Geometry: final body of the model. Coordinates: model frame, mm. A direction names the side the tool comes from. Round coordinates to 2 decimals unless told otherwise and drop trailing zeros. Write each loop counter-clockwise with the first axis right and the second up, starting at its lowest first coordinate (ties: lowest second). Pieces come first, ordered by that corner, then holes. Notation, with made-up numbers: M -1.5,67 L 36.5,67 A28 ccw 36.5,103 Z; hole C 1,-10.75 d7. An arc over 180 degrees is marked long. Use one line per item in the form item = value. Start each with the question number.
Item 1: Pull-direction query (Y, two-part tool) for faces 1 (the flat face through (-28.975, 8.916, 5.105)), 2 (the cylindrical face through (-23.116, 6.452, 0.105)), 3 (the flat face through (-27, 0, 2)), 4 (the cylindrical face through (23.116, 6.452, 0.105)); classes: pulls with the +Y half, pulls with the -Y half, needs draft (parallel to the pull), parting line crosses it, or undercut.
Item 2: Reachability of faces 5 (the flat face through (0, 22, -4.5)), 6 (the flat face through (-24.22, 8.84, 1.77)), 7 (the cylindrical face through (-17.81, 15.51, 4.05)), 8 (the flat face through (27, 0, 2)) from +Z, -Z, +X, -X, +Y, -Y: full face, straight path, thin tool, end or side. Return the list, or none.
Item 3: Ray query, probe 1 along Z at (x, y) = (14.5, 15.25); probe 2 along X at (y, z) = (1, 0); probe 3 along X at (y, z) = (5.5, 5). Return the intervals inside material, ascending.
Item 4: Section query B-B (x = 0). Return loops of the section in (y, z).
Item 5: Pin query (flat end, axial travel): pin 1 Ø3 at (y, z) = (5.5, -2.5) entering from -X; pin 2 Ø4.5 at (x, z) = (30.5, 2) entering from +Y; pin 3 Ø2 at (y, z) = (11, 0.5) entering from +X. Return the tip coordinate at first contact, or that it passes through.
Item 6: Section query A-A (z = -6). Return loops of the section in (x, y).
Item 7: Section query D-D (y = 22). Return loops of the section in (x, z), and give its area (3 significant figures).
Item 8: Section query C-C (y = 7.75). Return loops of the section in (x, z), and give its area (3 significant figures).
from build123d import *

# Parameters (mm, degrees)
SALIENTE_EXTRUIR1_DEPTH = 7.5
SALIENTE_EXTRUIR2_DEPTH = 7.5
CROQUIS3_R              = 2.25
CORTAR_EXTRUIR1_DEPTH   = 46.436769251
CROQUIS4_R              = 4.5
CORTAR_EXTRUIR2_DEPTH   = 44.789268092
CORTAR_EXTRUIR3_DEPTH   = 48.257274572
CORTAR_EXTRUIR4_DEPTH   = 15


with BuildPart() as part:
    # Croquis1 → Saliente-Extruir1 (new, symmetric)
    with BuildSketch(Plane.XY):
        with BuildLine():
            Line((-26, 0), (-21, 0))
            ThreePointArc((-21, 0), (0, 21), (21, 0))
            Line((21, 0), (26, 0))
            ThreePointArc((26, 0), (0, 26), (-26, 0))
        make_face()
    extrude(amount=SALIENTE_EXTRUIR1_DEPTH, both=True)

    # Croquis2 → Saliente-Extruir2 (add, symmetric)
    with BuildSketch(Plane.XY):
        with BuildLine():
            Line((26, 0), (36.5, 0))
            Line((36.5, 0), (36.5, 3))
            Line((36.5, 3), (21.236760582, 15))
            ThreePointArc((21.236760582, 15), (24.78059498, 7.869060455), (26, 0))
        make_face()
    saliente_extruir2 = extrude(amount=SALIENTE_EXTRUIR2_DEPTH, both=True)

    # Croquis3 → Cortar-Extruir1 (cut, through all)
    with BuildSketch(Plane.XZ):
        with Locations(Location((28.75, 0, 0), (0, 0, 270))):
            Circle(CROQUIS3_R)
    cortar_extruir1 = extrude(amount=-CORTAR_EXTRUIR1_DEPTH, mode=Mode.SUBTRACT)

    # Croquis4 → Cortar-Extruir2 (cut, through all)
    with BuildSketch(Plane(origin=(0, 3, 0), x_dir=(-1, 0, 0), z_dir=(0, -1, 0))):
        with Locations(Location((-28.75, 0, 0), (0, 0, 90))):
            Circle(CROQUIS4_R)
    cortar_extruir2 = extrude(amount=-CORTAR_EXTRUIR2_DEPTH, mode=Mode.SUBTRACT)

    # Simetría1: Saliente-Extruir2 across plane
    add(saliente_extruir2.mirror(Plane(origin=(0, 0, 0), x_dir=(0, 0, 1), z_dir=(1, 0, 0))))

    # Croquis6 → Cortar-Extruir3 (cut, through all)
    with BuildSketch(Plane.XY.offset(7.5)):
        with BuildLine():
            Line((30.510170652, 3.893065888), (22.898948379, 9.877029369))
            ThreePointArc((22.898948379, 9.877029369), (22.28692582, 9.881701061), (22.128900164, 9.290413206))
            ThreePointArc((22.128900164, 9.290413206), (23.12783497, 6.411181608), (23.753839647, 3.428571429))
            ThreePointArc((23.753839647, 3.428571429), (23.921384471, 3.122035527), (24.248711306, 3))
            Line((24.248711306, 3), (30.201141191, 3))
            ThreePointArc((30.201141191, 3), (30.673652007, 3.336496092), (30.510170652, 3.893065888))
        make_face()
    cortar_extruir3 = extrude(amount=-CORTAR_EXTRUIR3_DEPTH, mode=Mode.SUBTRACT)

    # Croquis8 → Cortar-Extruir4 (cut)
    with BuildSketch(Plane(origin=(0, 26, 0), x_dir=(1, 0, 0), z_dir=(0, 1, 0))):
        with BuildLine():
            Line((-16.736760582, -4.5), (16.736760582, -4.5))
            ThreePointArc((16.736760582, -4.5), (17.797420753, -4.060660172), (18.236760582, -3))
            Line((18.236760582, -3), (18.236760582, 3))
            ThreePointArc((18.236760582, 3), (17.797420753, 4.060660172), (16.736760582, 4.5))
            Line((16.736760582, 4.5), (-16.736760582, 4.5))
            ThreePointArc((-16.736760582, 4.5), (-17.797420753, 4.060660172), (-18.236760582, 3))
            Line((-18.236760582, 3), (-18.236760582, -3))
            ThreePointArc((-18.236760582, -3), (-17.797420753, -4.060660172), (-16.736760582, -4.5))
        make_face()
    extrude(amount=-CORTAR_EXTRUIR4_DEPTH, mode=Mode.SUBTRACT)

    # Simetría2: Cortar-Extruir1, Cortar-Extruir2, Cortar-Extruir3 across plane
    add(cortar_extruir1.mirror(Plane(origin=(0, 0, 0), x_dir=(0, 0, 1), z_dir=(1, 0, 0))), mode=Mode.SUBTRACT)
    add(cortar_extruir2.mirror(Plane(origin=(0, 0, 0), x_dir=(0, 0, 1), z_dir=(1, 0, 0))), mode=Mode.SUBTRACT)
    add(cortar_extruir3.mirror(Plane(origin=(0, 0, 0), x_dir=(0, 0, 1), z_dir=(1, 0, 0))), mode=Mode.SUBTRACT)


solid = part.part
Working result:
q1.face_1 = pulls with the +Y half
q1.face_2 = undercut
q1.face_3 = pulls with the -Y half
q1.face_4 = undercut
q2.face_5 = +Y, -Y
q2.face_6 = +Z, -Z
q2.face_7 = +Y
q2.face_8 = +Z, -Z, +X, -X, -Y
q3.probe_1 = -7.5 to -4.5, 4.5 to 7.5
q3.probe_2 = -36.5 to -31, -26.5 to -20.98, 20.98 to 26.5, 31 to 36.5
q3.probe_3 = -33.32 to -28.47, -23.36 to -20.27, 20.27 to 23.36, 28.47 to 33.32
q4.outline = M 21,-7.5 L 26,-7.5 L 26,-4.5 L 21,-4.5 Z; M 21,4.5 L 26,4.5 L 26,7.5 L 21,7.5 Z
q5.pin_1 = -35.23
q5.pin_2 = 7.9
q5.pin_3 = 24.51
q6.outline = M -36.5,0 L -21,0 A21 cw 21,0 L 36.5,0 L 36.5,3 L 21.24,15 A26 ccw -21.24,15 L -36.5,3 Z; hole M -30.51,3.89 A0.5 ccw -30.2,3 L -24.25,3 A0.5 ccw -23.75,3.43 A24 cw -22.13,9.29 A0.5 ccw -22.9,9.88 Z; hole M 22.13,9.29 A24 cw 23.75,3.43 A0.5 ccw 24.25,3 L 30.2,3 A0.5 ccw 30.51,3.89 L 22.9,9.88 A0.5 ccw Z
q7.outline = M -13.86,-7.5 L 13.86,-7.5 L 13.86,-4.5 L -13.86,-4.5 Z; M -13.86,4.5 L 13.86,4.5 L 13.86,7.5 L -13.86,7.5 Z
q7.area = 166 mm²
q8.outline = M -30.46,-7.5 L -25.6,-7.5 L -25.6,-3.22 A4.5 cw -30.46,-4.16 Z; M -30.46,4.16 A4.5 cw -25.6,3.22 L -25.6,7.5 L -30.46,7.5 Z; M -22.71,-7.5 L -19.52,-7.5 L -19.52,7.5 L -22.71,7.5 Z; M 19.52,-7.5 L 22.71,-7.5 L 22.71,7.5 L 19.52,7.5 Z; M 25.6,-7.5 L 30.46,-7.5 L 30.46,-4.16 A4.5 cw 25.6,-3.22 Z; M 25.6,3.22 A4.5 cw 30.46,4.16 L 30.46,7.5 L 25.6,7.5 Z
q8.area = 160 mm²
